```python
from build123d import *

# Parameters (mm, degrees)
BOX056_W                  = 10
BOX056_H                  = 4
BOX056_DEPTH              = 5.8
CYLINDER077_R             = 2.2
CYLINDER077_DEPTH         = 25
CYLINDER076_R             = 2.2
CYLINDER076_DEPTH         = 25
CYLINDER075_R             = 4
CYLINDER075_DEPTH         = 6
BOX055_W                  = 30
BOX055_H                  = 9.3
BOX055_DEPTH              = 13
FUSION042_ROLL_ANGLE      = 90
FUSION042_PLACEMENT_ANGLE = 90


with BuildPart() as quader035:
    # Box056 → Box056 (new body)
    with BuildSketch(Plane(origin=(-5, 8, 2), x_dir=(1, 0, 0), z_dir=(0, 0, 1))):
        with Locations((5, 2)):
            Rectangle(BOX056_W, BOX056_H)
    extrude(amount=BOX056_DEPTH)


with BuildPart() as zylinder066:
    # Cylinder077 → Cylinder077 (new body)
    with BuildSketch(Plane(origin=(-10, 12, 5), x_dir=(1, 0, 0), z_dir=(0, -1, 0))):
        Circle(CYLINDER077_R)
    extrude(amount=CYLINDER077_DEPTH)


with BuildPart() as zylinder065:
    # Cylinder076 → Cylinder076 (new body)
    with BuildSketch(Plane(origin=(10, 12, 5), x_dir=(1, 0, 0), z_dir=(0, -1, 0))):
        Circle(CYLINDER076_R)
    extrude(amount=CYLINDER076_DEPTH)


with BuildPart() as zylinder064:
    # Cylinder075 → Cylinder075 (new body)
    with BuildSketch(Plane.XY.offset(5.8)):
        Circle(CYLINDER075_R)
    extrude(amount=CYLINDER075_DEPTH)


with BuildPart() as y_drive_mount001:
    # Box055 → Box055 (new body)
    with BuildSketch(Plane(origin=(-15, 0, -2), x_dir=(1, 0, 0), z_dir=(0, 0, 1))):
        with Locations((15, 4.65)):
            Rectangle(BOX055_W, BOX055_H)
    extrude(amount=BOX055_DEPTH)

    # Cut084: cut Zylinder064
    add(zylinder064.part, mode=Mode.SUBTRACT)

    # Cut085: cut Zylinder065
    add(zylinder065.part, mode=Mode.SUBTRACT)

    # Cut086: cut Zylinder066
    add(zylinder066.part, mode=Mode.SUBTRACT)

    # Fusion042: union Quader035
    add(quader035.part)


with BuildPart() as y_drive_mount001_1:
    # Fusion042 roll: moved
    add(y_drive_mount001.part.rotate(Axis((0, 0, 0), (1, 0, 0)), FUSION042_ROLL_ANGLE))


with BuildPart() as y_drive_mount001_2:
    # Fusion042 placement: moved
    add(y_drive_mount001_1.part.moved(Location((-32.75, 18.85, 53.2))).rotate(Axis((-32.75, 18.85, 53.2), (0, 0, 1)), FUSION042_PLACEMENT_ANGLE))


solid = y_drive_mount001_2.part
```
Work out the finished part from the listing and answer in its coordinate system (mm). A direction names the side the tool comes from. Give positions to 0.01 mm unless a question says otherwise; leave off trailing zeros. Loops run counter-clockwise (first coordinate to the right, second up) from the corner with the lowest first, then second, coordinate; pieces in that order, holes last. Notation, with made-up numbers: (80.25, -9.5) -> (121.25, -9.5) arc R11 cw to (121.25, -2.5) -> close; hole circle Ø8 at (19, 51). An arc over 180 degrees is marked (long way). Write item = value, one per line. Start each with the question number.
(1) Find section D-D on x = -23.75. Give the vertices of the cut face in (y, z).
(2) The mould has two halves that part along Y. Classify faces 5 (the cylindrical face through (-29.7, 29.87, 57.92)), 6 (the flat face through (-28, 3.85, 58)), 7 (the flat face through (-28, 23.85, 64)), 8 (the cylindrical face through (-29.898, 8.373, 57.915)): +Y half, -Y half, draft (parallel to the pull), parting line (faces both ways), or undercut.
(3) Given pin 1 Ø0.8 at (x, z) = (-26.5, 63.5) entering from -Y; pin 2 Ø5 at (y, z) = (19, 54.5) entering from +X; pin 3 Ø0.8 at (y, z) = (21, 63.5) entering from -X, each flat-ended and moving along its own axis, determine where each tip first touches the part or whether it passes through.
(4) Find section A-A on y = 28.85. Give the vertices of the cut face in (x, z), and give its area (3 significant figures).
(5) Find section C-C on z = 56.5. Give the vertices of the cut face in (x, y), and give its area (3 significant figures).
(6) Which of the six approach directions +Z, -Z, +X, -X, +Y, -Y give full straight-line access (tool end or side, diameter ignored) to faces 1 (the flat face through (-24.95, 19, 64)), 2 (the flat face through (-30.75, 19, 64)), 3 (the flat face through (-26.95, 19, 55)), 4 (the flat face through (-28, 13.85, 64))?
(7) Find section B-B on x = -27.75. Give the vertices of the cut face in (y, z), and give its area (3 significant figures).
(8) Find the intervals of material crossed by probe 1 along Y at (x, z) = (-27.75, 59.25); probe 2 along X at (y, z) = (28.85, 56.25); probe 3 along Y at (x, z) = (-27, 61.75), in increasing order. Write a range as from..to.
From the geometry:
q1.outline = (3.85, 53.2) -> (14.85, 53.2) arc R4 cw to (22.85, 53.2) -> (33.85, 53.2) -> (33.85, 62.5) -> (3.85, 62.5) -> close
q2.face_5 = undercut
q2.face_6 = -Y half
q2.face_7 = +Y half
q2.face_8 = undercut
q3.pin_1 = 13.85
q3.pin_2 = -26.95
q3.pin_3 = -30.75
q4.outline = (-34.75, 53.2) -> (-29.95, 53.2) -> (-29.95, 62.5) -> (-34.75, 62.5) -> close; (-25.55, 53.2) -> (-21.75, 53.2) -> (-21.75, 62.5) -> (-25.55, 62.5) -> close
q4.area = 80.0 mm^2
q5.outline = (-34.75, 3.85) -> (-21.75, 3.85) -> (-21.75, 16.59) -> (-26.95, 16.59) -> (-26.95, 21.11) -> (-21.75, 21.11) -> (-21.75, 33.85) -> (-34.75, 33.85) -> close; hole circle Ø4.4 at (-27.75, 8.85); hole circle Ø4.4 at (-27.75, 28.85)
q5.area = 336 mm^2
q6.face_1 = +Z, +X, +Y, -Y
q6.face_2 = +Z, -X, +Y, -Y
q6.face_3 = -Z, +X
q6.face_4 = +Z, +X, -X, -Y
q7.outline = (3.85, 53.2) -> (6.65, 53.2) -> (6.65, 62.5) -> (3.85, 62.5) -> close; (11.05, 53.2) -> (26.65, 53.2) -> (26.65, 62.5) -> (23.85, 62.5) -> (23.85, 65.2) -> (13.85, 65.2) -> (13.85, 62.5) -> (11.05, 62.5) -> close; (31.05, 53.2) -> (33.85, 53.2) -> (33.85, 62.5) -> (31.05, 62.5) -> close
q7.area = 224 mm^2
q8.probe_1 = 3.85..6.65, 11.05..26.65, 31.05..33.85
q8.probe_2 = -34.75..-29.95, -25.55..-21.75
q8.probe_3 = 3.85..6.78, 10.92..26.78, 30.92..33.85
